CAD build for the part. Positions are in the model's coordinates, mm. A direction names the side the tool comes from. Round coordinates to 2 decimals unless told otherwise and drop trailing zeros. Loops run counter-clockwise (first coordinate to the right, second up) from the corner with the lowest first, then second, coordinate; pieces in that order, holes last.
from build123d import *

# Parameters (mm, degrees)
F0_R     = 7.5
F0_R_2   = 13.533
F1_DEPTH = 25
F2_DEPTH = 0.4
F3_DEPTH = 25


with BuildPart() as f1:
    # F0 (on Top) → F1 (new body)
    with BuildSketch(Plane.XY):
        with BuildLine():
            ThreePointArc((-28.885683, -42.552377), (-15.109618, -49.160827), (0, -51.430414))
            ThreePointArc((0, -51.430414), (15.109618, -49.160827), (28.885683, -42.552377))
            Line((28.885683, -42.552377), (22.292488, -35.519605))
            Line((22.292488, -35.519605), (30.606489, -28.667756))
            Line((30.606489, -28.667756), (37.815153, -34.858308))
            ThreePointArc((37.815153, -34.858308), (41.960361, -29.739125), (45.41727, -24.132116))
            Line((45.41727, -24.132116), (35.735177, -21.945261))
            Line((35.735177, -21.945261), (40.905213, -9.239094))
            Line((40.905213, -9.239094), (50.166693, -11.330947))
            ThreePointArc((50.166693, -11.330947), (51.099803, -5.82216), (51.429832, -0.24466))
            Line((51.429832, -0.24466), (41.922666, -1.042791))
            Line((41.922666, -1.042791), (40.863441, 9.422129))
            Line((40.863441, 9.422129), (50.346898, 10.5013))
            ThreePointArc((50.346898, 10.5013), (48.5709, 16.910209), (45.982751, 23.036363))
            Line((45.982751, 23.036363), (38.221147, 17.255182))
            Line((38.221147, 17.255182), (30.721983, 28.543951))
            Line((30.721983, 28.543951), (38.373263, 34.242958))
            ThreePointArc((38.373263, 34.242958), (33.412506, 39.09849), (27.843076, 43.241769))
            Line((27.843076, 43.241769), (23.645456, 34.633651))
            Line((23.645456, 34.633651), (11.384548, 40.360741))
            Line((11.384548, 40.360741), (15.600841, 49.007155))
            ThreePointArc((15.600841, 49.007155), (7.89396, 50.820988), (0, 51.430414))
            ThreePointArc((0, 51.430414), (-7.89396, 50.820988), (-15.600841, 49.007155))
            Line((-15.600841, 49.007155), (-11.384548, 40.360741))
            Line((-11.384548, 40.360741), (-23.645456, 34.633651))
            Line((-23.645456, 34.633651), (-27.843076, 43.241769))
            ThreePointArc((-27.843076, 43.241769), (-33.412506, 39.09849), (-38.373263, 34.242958))
            Line((-38.373263, 34.242958), (-30.721983, 28.543951))
            Line((-30.721983, 28.543951), (-38.221147, 17.255182))
            Line((-38.221147, 17.255182), (-45.982751, 23.036363))
            ThreePointArc((-45.982751, 23.036363), (-48.5709, 16.910209), (-50.346898, 10.5013))
            Line((-50.346898, 10.5013), (-40.863441, 9.422129))
            Line((-40.863441, 9.422129), (-41.922666, -1.042791))
            Line((-41.922666, -1.042791), (-51.429832, -0.24466))
            ThreePointArc((-51.429832, -0.24466), (-51.099803, -5.82216), (-50.166693, -11.330947))
            Line((-50.166693, -11.330947), (-40.905213, -9.239094))
            Line((-40.905213, -9.239094), (-35.735177, -21.945261))
            Line((-35.735177, -21.945261), (-45.41727, -24.132116))
            ThreePointArc((-45.41727, -24.132116), (-41.960361, -29.739125), (-37.815153, -34.858308))
            Line((-37.815153, -34.858308), (-30.606489, -28.667756))
            Line((-30.606489, -28.667756), (-22.292488, -35.519605))
            Line((-22.292488, -35.519605), (-28.885683, -42.552377))
        make_face()
        with Locations((-25.715207, 0)):
            Circle(F0_R, mode=Mode.SUBTRACT)
        with Locations((0, -25.715207)):
            Circle(F0_R, mode=Mode.SUBTRACT)
        Circle(F0_R_2, mode=Mode.SUBTRACT)
        with Locations((25.715207, -2.612802)):
            Circle(F0_R, mode=Mode.SUBTRACT)
        with Locations((0, 32.481707)):
            Circle(F0_R, mode=Mode.SUBTRACT)
    extrude(amount=F1_DEPTH)

    # F0 (on Top) → F2 (cut)
    with BuildSketch(Plane.XY):
        Circle(F0_R_2)
    extrude(amount=-F2_DEPTH, mode=Mode.SUBTRACT)

    # F0 (on Top) → F3 (cut)
    with BuildSketch(Plane.XY):
        with Locations((0, 32.481707)):
            Circle(F0_R)
        with Locations((-25.715207, 0)):
            Circle(F0_R)
        with Locations((25.715207, -2.612802)):
            Circle(F0_R)
        with Locations((0, -25.715207)):
            Circle(F0_R)
    extrude(amount=-F3_DEPTH, mode=Mode.SUBTRACT)


solid = f1.part
Item 1: Wall check: L1, parallel to Y at x = -31.5, z = 5.75; L2, parallel to Y at x = 38, z = 15.25; L3, parallel to Y at x = -6, z = 23.75. Give the ranges that are in metal, low to high.
Verdict:
L1: y = -29.44 to -4.77, 4.77 to 27.37, 29.12 to 40.66
L2: y = -34.66 to -22.46, -16.38 to 17.59, 33.96 to 34.66
L3: y = -51.08 to -30.22, -21.22 to -12.13, 12.13 to 27.98, 36.98 to 51.08
Item 2: Cut at A-A (x = 21). List the corners of the cut face in (y, z).
Verdict:
outline: (-46.95, 0) - (-8.45, 0) - (-8.45, 25) - (-46.95, 25) - close; (3.22, 0) - (35.87, 0) - (35.87, 25) - (3.22, 25) - close
Item 3: Cut at D-D (z = 15.5). State how many separate pieces and enclosed holes the cut face has, plus the area to 3 significant figures.
Verdict:
separate pieces: 1
enclosed holes: 5
area: 5,790 mm2
Item 4: 3-axis set-ups, long thin cutter, end or side, ignore diameter. For faces 1 (the flat face through (-34.6, 31.43, 12.32)), 2 (the flat face through (17.601, 37.457, 12.325)), 3 (the flat face through (45.539, 9.954, 12.325)): which of +Z, -Z, +X, -X, +Y, -Y reach the whole face in a straight line?
Verdict:
face 1: +Z, -Z, -X
face 2: +Z, -Z
face 3: +Z, -Z, +X
Item 5: Cut at B-B (y = -31). List the corners of the cut face in (x, z).
Verdict:
outline: (-41.04, 0) - (-33.32, 0) - (-33.32, 25) - (-41.04, 25) - close; (-27.78, 0) - (-5.32, 0) - (-5.32, 25) - (-27.78, 25) - close; (5.32, 0) - (27.78, 0) - (27.78, 25) - (5.32, 25) - close; (33.32, 0) - (41.04, 0) - (41.04, 25) - (33.32, 25) - close
Item 6: Mould opens along Y. For faces 4 (the flat face through (-26.508, -32.046, 12.325)), 5 (the flat face through (-34.261, -31.806, 12.325)), 6 (the cylindrical face through (33.486, 39.035, 12.325)) say: released by +Y, released by -Y, zero draft, split by the parting line, or undercut.
Verdict:
face 4: undercut
face 5: released by -Y
face 6: released by +Y
Item 7: Flat gauge pins, fed straight in: P1, Ø3, axis at x = -9, z = 15.5, coming from the +Y side; P2, Ø6, axis at x = 16.5, y = -5, coming from the -Z side; P3, Ø12, axis at x = -24, z = 17, coming from the -Y side; P4, Ø9, axis at x = 0, y = -25.72, coming from the +Z side. Where does each tip first touch, or does it go through?
Verdict:
P1: stops at y = 50.88
P2: stops at z = 0
P3: stops at y = -48.18
P4: passes through
Item 8: Cut at C-C (x = 10). List the corners of the cut face in (y, z), plus the area to 3 significant figures.
Verdict:
outline: (-50.45, 0) - (-9.12, 0) - (-9.12, 25) - (-50.45, 25) - close; (9.12, 0) - (50.45, 0) - (50.45, 25) - (9.12, 25) - close
area: 2,070 mm2
